Verification items for the finished model (mm, model axes). A direction names the side the tool comes from. Round coordinates to 2 decimals unless told otherwise and drop trailing zeros. Write each loop counter-clockwise with the first axis right and the second up, starting at its lowest first coordinate (ties: lowest second). Pieces come first, ordered by that corner, then holes. Notation, with made-up numbers: (30.25, 19) - (45.25, 19) arc R36 ccw to (45.25, 53) - close; hole circle Ø8 at (-23, 78). An arc over 180 degrees is marked (long way). Write each question's results on one line, items separated by ' | '.
```python
from build123d import *

# Parameters (mm, degrees)
BOSS_EXTRUDE1_DEPTH = 500
CUT_EXTRUDE1_DEPTH  = 570.957034721
SKETCH3_W           = 88.9
SKETCH3_H           = 25.400000016
BOSS_EXTRUDE2_DEPTH = 1
SKETCH4_W           = 88.9
SKETCH4_H           = 25.40000001
BOSS_EXTRUDE3_DEPTH = 1
FILLET1_R           = 109.330995043


with BuildPart() as part:
    # Sketch1 → Boss-Extrude1 (new body)
    with BuildSketch(Plane(origin=(-250, 0, 0), x_dir=(0, -1, 0), z_dir=(-1, 0, 0))):
        Polygon((106.330251065, -252.08113602), (106.330251065, 0), (-25.401284991, 0), (-25.401284991, -67.909513139), (80.930251056, -252.08113602), align=None)
    extrude(amount=-BOSS_EXTRUDE1_DEPTH)

    # Sketch2 → Cut-Extrude1 (cut, through all)
    with BuildSketch(Plane(origin=(250, 0, 0), x_dir=(0, 0, -1), z_dir=(1, 0, 0))):
        Polygon((183.427309509, -106.33025104), (77.097058469, 0), (0, 0), (0, -106.33025104), align=None)
    extrude(amount=-CUT_EXTRUDE1_DEPTH, mode=Mode.SUBTRACT)

    # Sketch3 → Boss-Extrude2 (add)
    with BuildSketch(Plane.XZ):
        with Locations((-95.25, -19.110677533)):
            Rectangle(SKETCH3_W, SKETCH3_H)
    extrude(amount=BOSS_EXTRUDE2_DEPTH)

    # Sketch4 → Boss-Extrude3 (add)
    with BuildSketch(Plane.XZ):
        with Locations((95.25, -19.110677536)):
            Rectangle(SKETCH4_W, SKETCH4_H)
    extrude(amount=BOSS_EXTRUDE3_DEPTH)

    # Fillet1
    fillet1_edges = [part.edges().sort_by_distance(p)[0] for p in [
        (0, 0, -77.097058469),
    ]]
    fillet(fillet1_edges, radius=FILLET1_R - 0.0001)  # a hair under: the kernel refuses the full size


solid = part.part
```
(1) Section check A-A (z = -23). Record the cut outline in (x, y).
Answer:
outline: (-250, 0) - (-139.7, 0) - (-139.7, -1) - (-50.8, -1) - (-50.8, 0) - (50.8, 0) - (50.8, -1) - (139.7, -1) - (139.7, 0) - (250, 0) - (250, 25.4) - (-250, 25.4) - close
(2) Thickness scan on L1, parallel to Y at x = 11, z = -25; L2, parallel to Y at x = 50.5, z = -47; L3, parallel to Z at x = 48, y = -38. Record the ranges inside material, lowest first.
Answer:
L1: 0 to 25.4 | L2: -1.06 to 25.4 | L3: -177.72 to -115.1
(3) Set-up check for faces 1 (the flat face through (-4, 25.401, -33)), 2 (the flat face through (-96, -1, -19)): record each of +Z, -Z, +X, -X, +Y, -Y from which the full face is reachable in a straight line by a thin tool's end or side.
Answer:
face 1: +Z, -Z, +X, -X, +Y | face 2: +Z, +X, -X, -Y
(4) Section check B-B (x = -148). Record the cut outline in (y, z).
Answer:
outline: (-106.33, -252.08) - (-80.93, -252.08) - (25.4, -67.91) - (25.4, 0) - (0, 0) - (0, -31.81) arc R109.33 cw to (-32.02, -109.12) - (-106.33, -183.43) - close
(5) Section check C-C (y = -41). Record the cut outline in (x, z), plus the area to 3 significant figures.
Answer:
outline: (-250, -182.92) - (250, -182.92) - (250, -118.1) - (-250, -118.1) - close | area: 32,400 mm2
(6) Go/stop test with flat-tipped pins: pin 1 Ø3 at (x, y) = (-10.5, -75.5) entering from +Z; pin 2 Ø1.1 at (x, y) = (-111, -0.5) entering from +Z; pin 3 Ø0.8 at (x, y) = (78, -0.5) entering from -Z; pin 4 Ø1.5 at (x, y) = (-34.5, 9.5) entering from -Z. Record where each tip stops, or that it passes through.
Answer:
pin 1: z = -151.1 | pin 2: z = 0 | pin 3: z = -113.46 | pin 4: z = -96.75
